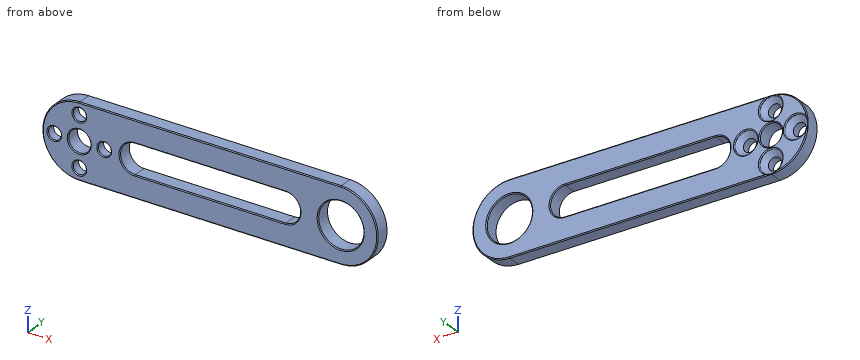
```python
from build123d import *

# Parameters (mm, degrees)
SKETCH1_R                                      = 1.75
SKETCH1_R_2                                    = 3
SKETCH1_R_3                                    = 6.125
BOSS_EXTRUDE1_DEPTH                            = 2
CSK_FOR_M3_FLAT_HEAD_MACHINE_SCREW2_AT_2_COUNT = 2
CSK_FOR_M3_FLAT_HEAD_MACHINE_SCREW2_AT_2_PITCH = 9.545941546
CSK_FOR_M3_FLAT_HEAD_MACHINE_SCREW2_AT_3_COUNT = 2
CSK_FOR_M3_FLAT_HEAD_MACHINE_SCREW2_AT_3_PITCH = 13.5
CSK_FOR_M3_FLAT_HEAD_MACHINE_SCREW2_AT_4_COUNT = 2
CSK_FOR_M3_FLAT_HEAD_MACHINE_SCREW2_AT_4_PITCH = 9.545941546
CHAMFER1_SIZE                                  = 0.25


with BuildPart() as part:
    # Sketch1 → Boss-Extrude1 (new, symmetric)
    with BuildSketch(Plane(origin=(0, 0, 0), x_dir=(1, 0, 0), z_dir=(0, 1, 0))):
        with BuildLine():
            Line((0, 10), (70.71, 10))
            ThreePointArc((70.71, 10), (80.71, 0), (70.71, -10))
            Line((70.71, -10), (0, -10))
            ThreePointArc((0, -10), (-10, 0), (0, 10))
        make_face()
        with Locations(Location((0, 6.75, 0), (0, 0, 270))):
            Circle(SKETCH1_R, mode=Mode.SUBTRACT)
        with Locations(Location((6.75, 0, 0), (0, 0, 270))):
            Circle(SKETCH1_R, mode=Mode.SUBTRACT)
        with Locations(Location((0, -6.75, 0), (0, 0, 270))):
            Circle(SKETCH1_R, mode=Mode.SUBTRACT)
        with Locations(Location((-6.75, 0, 0), (0, 0, 270))):
            Circle(SKETCH1_R, mode=Mode.SUBTRACT)
        with Locations(Location((0, 0, 0), (0, 0, 270))):
            Circle(SKETCH1_R_2, mode=Mode.SUBTRACT)
        with Locations(Location((70.71, 0, 0), (0, 0, 270))):
            Circle(SKETCH1_R_3, mode=Mode.SUBTRACT)
        with BuildLine():
            Line((15, 4), (55.71, 4))
            ThreePointArc((55.71, 4), (59.71, 0), (55.71, -4))
            Line((55.71, -4), (15, -4))
            ThreePointArc((15, -4), (11, 0), (15, 4))
        make_face(mode=Mode.SUBTRACT)
    extrude(amount=BOSS_EXTRUDE1_DEPTH, both=True)

    # Sketch3 → CSK for M3 Flat Head Machine Screw2 (revolve, cut)
    with BuildSketch(Plane(origin=(0, 2, -6.75), x_dir=(0, 0, 1), z_dir=(1, 0, 0))):
        Polygon((0, 0), (0, 4), (1.75, 4), (1.75, 1.65), (3.1, 0.3), (3.1, 0), align=None)
    csk_for_m3_flat_head_machine_screw2 = revolve(axis=Axis((0, 8.35, -6.75), (0, -1, 0)), mode=Mode.SUBTRACT)

    # CSK for M3 Flat Head Machine Screw2 at 2: CSK for M3 Flat Head Machine Screw2 ×2
    with Locations(*[Vector(0.7071067811865476, 0, 0.7071067811865476) * (i * CSK_FOR_M3_FLAT_HEAD_MACHINE_SCREW2_AT_2_PITCH) for i in range(1, CSK_FOR_M3_FLAT_HEAD_MACHINE_SCREW2_AT_2_COUNT)]):
        add(csk_for_m3_flat_head_machine_screw2, mode=Mode.SUBTRACT)

    # CSK for M3 Flat Head Machine Screw2 at 3: CSK for M3 Flat Head Machine Screw2 ×2
    with Locations(*[(0, 0, i * CSK_FOR_M3_FLAT_HEAD_MACHINE_SCREW2_AT_3_PITCH) for i in range(1, CSK_FOR_M3_FLAT_HEAD_MACHINE_SCREW2_AT_3_COUNT)]):
        add(csk_for_m3_flat_head_machine_screw2, mode=Mode.SUBTRACT)

    # CSK for M3 Flat Head Machine Screw2 at 4: CSK for M3 Flat Head Machine Screw2 ×2
    with Locations(*[Vector(-0.7071067811865476, 0, 0.7071067811865476) * (i * CSK_FOR_M3_FLAT_HEAD_MACHINE_SCREW2_AT_4_PITCH) for i in range(1, CSK_FOR_M3_FLAT_HEAD_MACHINE_SCREW2_AT_4_COUNT)]):
        add(csk_for_m3_flat_head_machine_screw2, mode=Mode.SUBTRACT)

    # Chamfer1
    # the kernel refuses this chamfer: 0.25 mm, written as the material it takes off along each edge
    with BuildSketch(Plane(origin=(0, -2, -6.75), x_dir=(0, 0, 1), z_dir=(-1, 0, 0))) as chamfer1_piece_1:
        Polygon((1.75 + CHAMFER1_SIZE, 0), (1.75, CHAMFER1_SIZE), (1.75, 0), align=None)
    revolve(axis=Axis((0, -2, -6.75), (0, 1, 0)), mode=Mode.SUBTRACT)
    with BuildSketch(Plane(origin=(70.71, 2, 0), x_dir=(0, 0, -1), z_dir=(-1, 0, 0))) as chamfer1_piece_2:
        Polygon((10, CHAMFER1_SIZE), (10 - CHAMFER1_SIZE, 0), (10, 0), align=None)
    revolve(axis=Axis((70.71, 2, 0), (0, -1, 0)), revolution_arc=180, mode=Mode.SUBTRACT)
    with BuildSketch(Plane(origin=(6.75, -2, 0), x_dir=(0, 0, 1), z_dir=(-1, 0, 0))) as chamfer1_piece_3:
        Polygon((1.75 + CHAMFER1_SIZE, 0), (1.75, CHAMFER1_SIZE), (1.75, 0), align=None)
    revolve(axis=Axis((6.75, -2, 0), (0, 1, 0)), mode=Mode.SUBTRACT)
    with BuildSketch(Plane(origin=(0, 2, -10), x_dir=(0, -0.9996219169112968, -0.027495876610589075), z_dir=(1, 0, 0)), Plane(origin=(70.71, -2, 10), x_dir=(0, -0.02749587661058555, -0.9996219169112968), z_dir=(-1, 0, 0))) as chamfer1_piece_4:
        Polygon((CHAMFER1_SIZE * 0.999621916911, -CHAMFER1_SIZE * 0.0274958766106), (-CHAMFER1_SIZE * 0.0274958766106, -CHAMFER1_SIZE * 0.999621916911), (0, 0), align=None)
    extrude(amount=70.71, mode=Mode.SUBTRACT)
    with BuildSketch(Plane(origin=(0, -2, 6.75), x_dir=(0, 0, 1), z_dir=(-1, 0, 0))) as chamfer1_piece_5:
        Polygon((1.75 + CHAMFER1_SIZE, 0), (1.75, CHAMFER1_SIZE), (1.75, 0), align=None)
    revolve(axis=Axis((0, -2, 6.75), (0, 1, 0)), mode=Mode.SUBTRACT)
    with BuildSketch(Plane(origin=(-6.75, -2, 0), x_dir=(0, 0, 1), z_dir=(-1, 0, 0))) as chamfer1_piece_6:
        Polygon((1.75 + CHAMFER1_SIZE, 0), (1.75, CHAMFER1_SIZE), (1.75, 0), align=None)
    revolve(axis=Axis((-6.75, -2, 0), (0, 1, 0)), mode=Mode.SUBTRACT)
    with BuildSketch(Plane(origin=(0, -2, 0), x_dir=(0, 0, 1), z_dir=(-1, 0, 0))) as chamfer1_piece_7:
        Polygon((3 + CHAMFER1_SIZE, 0), (3, CHAMFER1_SIZE), (3, 0), align=None)
    revolve(axis=Axis((0, -2, 0), (0, 1, 0)), mode=Mode.SUBTRACT)
    with BuildSketch(Plane(origin=(0, 2, 0), x_dir=(0, 0, 1), z_dir=(-1, 0, 0))) as chamfer1_piece_8:
        Polygon((3 + CHAMFER1_SIZE, 0), (3, -CHAMFER1_SIZE), (3, 0), align=None)
    revolve(axis=Axis((0, 2, 0), (0, 1, 0)), mode=Mode.SUBTRACT)
    with BuildSketch(Plane(origin=(70.71, -2, 0), x_dir=(0, 0, 1), z_dir=(-1, 0, 0))) as chamfer1_piece_9:
        Polygon((6.125 + CHAMFER1_SIZE, 0), (6.125, CHAMFER1_SIZE), (6.125, 0), align=None)
    revolve(axis=Axis((70.71, -2, 0), (0, 1, 0)), mode=Mode.SUBTRACT)
    with BuildSketch(Plane(origin=(70.71, 2, 0), x_dir=(0, 0, 1), z_dir=(-1, 0, 0))) as chamfer1_piece_10:
        Polygon((6.125 + CHAMFER1_SIZE, 0), (6.125, -CHAMFER1_SIZE), (6.125, 0), align=None)
    revolve(axis=Axis((70.71, 2, 0), (0, 1, 0)), mode=Mode.SUBTRACT)
    with BuildSketch(Plane(origin=(15, -2, 0), x_dir=(0, 0, 1), z_dir=(1, 0, 0))) as chamfer1_piece_11:
        Polygon((4 + CHAMFER1_SIZE, 0), (4, -CHAMFER1_SIZE), (4, 0), align=None)
    revolve(axis=Axis((15, -2, 0), (0, -1, 0)), revolution_arc=180, mode=Mode.SUBTRACT)
    with BuildSketch(Plane(origin=(55.71, -2, 4), x_dir=(0, -0.0274958766105856, 0.9996219169112968), z_dir=(-1, 0, 0)), Plane(origin=(15, -2, -4), x_dir=(0, -0.027495876610585647, -0.9996219169112968), z_dir=(1, 0, 0))) as chamfer1_piece_12:
        Polygon((CHAMFER1_SIZE * 0.999621916911, CHAMFER1_SIZE * 0.0274958766106), (-CHAMFER1_SIZE * 0.0274958766106, CHAMFER1_SIZE * 0.999621916911), (0, 0), align=None)
    extrude(amount=40.71, mode=Mode.SUBTRACT)
    with BuildSketch(Plane(origin=(55.71, -2, 0), x_dir=(0, 0, -1), z_dir=(-1, 0, 0))) as chamfer1_piece_13:
        Polygon((4 + CHAMFER1_SIZE, 0), (4, -CHAMFER1_SIZE), (4, 0), align=None)
    revolve(axis=Axis((55.71, -2, 0), (0, -1, 0)), revolution_arc=180, mode=Mode.SUBTRACT)
    with BuildSketch(Plane(origin=(15, 2, 0), x_dir=(0, 0, 1), z_dir=(1, 0, 0))) as chamfer1_piece_14:
        Polygon((4 + CHAMFER1_SIZE, 0), (4, CHAMFER1_SIZE), (4, 0), align=None)
    revolve(axis=Axis((15, 2, 0), (0, -1, 0)), revolution_arc=180, mode=Mode.SUBTRACT)
    with BuildSketch(Plane(origin=(55.71, 2, 4), x_dir=(0, 0.0274958766105856, 0.9996219169112968), z_dir=(-1, 0, 0)), Plane(origin=(15, 2, -4), x_dir=(0, 0.027495876610585647, -0.9996219169112968), z_dir=(1, 0, 0))) as chamfer1_piece_15:
        Polygon((CHAMFER1_SIZE * 0.999621916911, -CHAMFER1_SIZE * 0.0274958766106), (-CHAMFER1_SIZE * 0.0274958766106, -CHAMFER1_SIZE * 0.999621916911), (0, 0), align=None)
    extrude(amount=40.71, mode=Mode.SUBTRACT)
    with BuildSketch(Plane(origin=(55.71, 2, 0), x_dir=(0, 0, -1), z_dir=(-1, 0, 0))) as chamfer1_piece_16:
        Polygon((4 + CHAMFER1_SIZE, 0), (4, CHAMFER1_SIZE), (4, 0), align=None)
    revolve(axis=Axis((55.71, 2, 0), (0, -1, 0)), revolution_arc=180, mode=Mode.SUBTRACT)
    with BuildSketch(Plane(origin=(0, 2, 0), x_dir=(0, 0, 1), z_dir=(1, 0, 0))) as chamfer1_piece_17:
        Polygon((10, CHAMFER1_SIZE), (10 - CHAMFER1_SIZE, 0), (10, 0), align=None)
    revolve(axis=Axis((0, 2, 0), (0, -1, 0)), revolution_arc=180, mode=Mode.SUBTRACT)
    with BuildSketch(Plane(origin=(0, -2, -10), x_dir=(0, 0.9996219169112968, -0.027495876610589075), z_dir=(1, 0, 0)), Plane(origin=(70.71, 2, 10), x_dir=(0, 0.02749587661058555, -0.9996219169112968), z_dir=(-1, 0, 0))) as chamfer1_piece_18:
        Polygon((CHAMFER1_SIZE * 0.999621916911, CHAMFER1_SIZE * 0.0274958766106), (-CHAMFER1_SIZE * 0.0274958766106, CHAMFER1_SIZE * 0.999621916911), (0, 0), align=None)
    extrude(amount=70.71, mode=Mode.SUBTRACT)
    with BuildSketch(Plane(origin=(70.71, -2, 0), x_dir=(0, 0, -1), z_dir=(-1, 0, 0))) as chamfer1_piece_19:
        Polygon((10 - CHAMFER1_SIZE, 0), (10, -CHAMFER1_SIZE), (10, 0), align=None)
    revolve(axis=Axis((70.71, -2, 0), (0, -1, 0)), revolution_arc=180, mode=Mode.SUBTRACT)
    with BuildSketch(Plane(origin=(-6.75, 2, 0), x_dir=(0, 0, 1), z_dir=(1, 0, 0))) as chamfer1_piece_20:
        Polygon((3.1 + CHAMFER1_SIZE, 0), (3.1, CHAMFER1_SIZE), (3.1, 0), align=None)
    revolve(axis=Axis((-6.75, 2, 0), (0, -1, 0)), mode=Mode.SUBTRACT)
    with BuildSketch(Plane(origin=(0, -2, 0), x_dir=(0, 0, 1), z_dir=(1, 0, 0))) as chamfer1_piece_21:
        Polygon((10, -CHAMFER1_SIZE), (10 - CHAMFER1_SIZE, 0), (10, 0), align=None)
    revolve(axis=Axis((0, -2, 0), (0, -1, 0)), revolution_arc=180, mode=Mode.SUBTRACT)
    with BuildSketch(Plane(origin=(0, 2, 6.75), x_dir=(0, 0, 1), z_dir=(1, 0, 0))) as chamfer1_piece_22:
        Polygon((3.1 + CHAMFER1_SIZE, 0), (3.1, CHAMFER1_SIZE), (3.1, 0), align=None)
    revolve(axis=Axis((0, 2, 6.75), (0, -1, 0)), mode=Mode.SUBTRACT)
    with BuildSketch(Plane(origin=(6.75, 2, 0), x_dir=(0, 0, 1), z_dir=(1, 0, 0))) as chamfer1_piece_23:
        Polygon((3.1 + CHAMFER1_SIZE, 0), (3.1, CHAMFER1_SIZE), (3.1, 0), align=None)
    revolve(axis=Axis((6.75, 2, 0), (0, -1, 0)), mode=Mode.SUBTRACT)
    with BuildSketch(Plane(origin=(0, 2, -6.75), x_dir=(0, 0, 1), z_dir=(1, 0, 0))) as chamfer1_piece_24:
        Polygon((3.1 + CHAMFER1_SIZE, 0), (3.1, CHAMFER1_SIZE), (3.1, 0), align=None)
    revolve(axis=Axis((0, 2, -6.75), (0, -1, 0)), mode=Mode.SUBTRACT)


solid = part.part
```
Could you check a few things on this model? Use its own coordinates, in mm. Round coordinates to 2 decimals unless told otherwise and drop trailing zeros. Order: outer loops, then holes, each group sorted by start corner. A loop starts at its lowest first (then second) coordinate and runs counter-clockwise, first axis right, second up. Notation, with made-up numbers: M 79.5,34.25 L 113.5,34.25 A31 cw 113.5,73.25 Z; hole C 22,-19.75 d5. An arc over 180 degrees is marked long. One line per question, with ' | ' between items. Start each with the question number.
(1) Please list where these lines run through material, in increasing order: line 1 along Z through (x, y) = (16, -0.35); line 2 along X through (y, z) = (0.1, 0) (3 decimals); line 3 along X through (y, z) = (-1.8, -1.25).
(2) For P1, Ø3.5, axis at x = 0, z = 0, coming from the +Y side; P2, Ø4, axis at x = -6.75, z = 0, coming from the +Y side, each with a flat end and sliding along its axis, tell me the tip position at first contact or that it passes through.
(3) Suppose I cut it at A-A on x = 53. List the corners of the cut face in (y, z) for me.
Geometry results:
1) line 1: -10 to -4, 4 to 10 | line 2: -10 to -8.5, -5 to -3, 3 to 5, 8.5 to 11, 59.71 to 64.585, 76.835 to 80.71 | line 3: -9.87 to -8.05, -5.45 to -2.78, 2.78 to 5.45, 8.05 to 11.15, 59.56 to 64.66, 76.76 to 80.58
2) P1: through | P2: y = 0.6
3) outline: M -2,-9.75 L -1.75,-10 L 1.75,-10 L 2,-9.75 L 2,-4.25 L 1.75,-4 L -1.75,-4 L -2,-4.25 Z; M -2,4.25 L -1.75,4 L 1.75,4 L 2,4.25 L 2,9.75 L 1.75,10 L -1.75,10 L -2,9.75 Z
